Verification items for the finished model (mm, model axes). Round coordinates to 2 decimals unless told otherwise and drop trailing zeros. Order: outer loops, then holes, each group sorted by start corner. A loop starts at its lowest first (then second) coordinate and runs counter-clockwise, first axis right, second up. Notation, with made-up numbers: (-27, 8.25) -> (0, 8.25) arc R25 ccw to (0, 40.25) -> close; hole circle Ø10 at (4, 57). An arc over 180 degrees is marked (long way). Put each result on its own line as item: value.
from build123d import *

# Parameters (mm, degrees)
SKETCH1_R           = 2
SKETCH1_R_2         = 0.75
SKETCH1_R_3         = 0.74964
SKETCH1_W           = 9
SKETCH1_H           = 2.000000357
SKETCH1_W_2         = 5
SKETCH1_H_2         = 2
SKETCH1_W_3         = 8
SKETCH1_H_3         = 6.000000353
SKETCH1_H_4         = 4
SKETCH1_W_4         = 6.000000352
BOSS_EXTRUDE1_DEPTH = 4


with BuildPart() as part:
    # Sketch1 → Boss-Extrude1 (new body)
    with BuildSketch(Plane.XY):
        with BuildLine():
            Line((-12.978641063, -17.999999648), (-12.978641063, -24))
            Line((-12.978641063, -24), (23.021361236, -24))
            Line((23.021361236, -24), (23.021361236, -17.999999648))
            ThreePointArc((23.021361236, -17.999999648), (32.577630228, -15.139859344), (38.991305368, -7.5))
            ThreePointArc((38.991305368, -7.5), (45.219254131, 9.097839331), (47.3354431, 26.698900677))
            ThreePointArc((47.3354431, 26.698900677), (46.554459277, 46.942107237), (44.216150624, 67.064971353))
            Line((44.216150624, 67.064971353), (28.143849376, 69.095028647))
            Line((28.143849376, 69.095028647), (26.638766331, 75.523635508))
            Line((26.638766331, 75.523635508), (10.441233669, 75.806364492))
            Line((10.441233669, 75.806364492), (8.1, 82.51))
            Line((8.1, 82.51), (-8.1, 82.51))
            Line((-8.1, 82.51), (-14.491235706, 82.281481113))
            Line((-14.491235706, 82.281481113), (-30.688764294, 81.998518887))
            ThreePointArc((-30.688764294, 81.998518887), (-37.914532987, 47.276776451), (-37.052658257, 11.821617405))
            ThreePointArc((-37.052658257, 11.821617405), (-29.143237496, -6.421257936), (-12.978641063, -17.999999648))
        make_face()
        with Locations((38.147341743, 11.821617405)):
            Circle(SKETCH1_R, mode=Mode.SUBTRACT)
        with Locations((-14, -9.124358764)):
            Circle(SKETCH1_R, mode=Mode.SUBTRACT)
        with Locations((-5.25, 80.01)):
            Circle(SKETCH1_R_2, mode=Mode.SUBTRACT)
        with Locations((-31.681501662, 43.456405989)):
            Circle(SKETCH1_R, mode=Mode.SUBTRACT)
        with Locations((5.25, 80.01)):
            Circle(SKETCH1_R_2, mode=Mode.SUBTRACT)
        with Locations((5.25, 74.01)):
            Circle(SKETCH1_R_2, mode=Mode.SUBTRACT)
        with Locations((-5.25, 74.01)):
            Circle(SKETCH1_R_2, mode=Mode.SUBTRACT)
        with Locations((-27.795567347, 79.548639007)):
            Circle(SKETCH1_R_2, mode=Mode.SUBTRACT)
        with Locations((-17.297097199, 79.732041708)):
            Circle(SKETCH1_R_2, mode=Mode.SUBTRACT)
        with Locations((-27.690766522, 73.549554345)):
            Circle(SKETCH1_R_2, mode=Mode.SUBTRACT)
        with Locations((-17.192296374, 73.732957046)):
            Circle(SKETCH1_R_2, mode=Mode.SUBTRACT)
        with Locations((23.640854945, 67.074669457)):
            Circle(SKETCH1_R_2, mode=Mode.SUBTRACT)
        with Locations((13.142454146, 67.257919725)):
            Circle(SKETCH1_R_2, mode=Mode.SUBTRACT)
        with Locations((23.745569383, 73.073755628)):
            Circle(SKETCH1_R_2, mode=Mode.SUBTRACT)
        with Locations((13.247168584, 73.257005896)):
            Circle(SKETCH1_R_2, mode=Mode.SUBTRACT)
        with Locations((29.906230336, 60.30489137)):
            Circle(SKETCH1_R_3, mode=Mode.SUBTRACT)
        with Locations((41.075335698, 64.94181766)):
            Circle(SKETCH1_R_3, mode=Mode.SUBTRACT)
        with Locations((30.658103408, 66.257595536)):
            Circle(SKETCH1_R_3, mode=Mode.SUBTRACT)
        with Locations((40.323462626, 58.989113494)):
            Circle(SKETCH1_R_3, mode=Mode.SUBTRACT)
        with Locations((0, 77.509999822)):
            Rectangle(SKETCH1_W, SKETCH1_H, mode=Mode.SUBTRACT)
        Polygon((-9.666, 24.072257636), (-9.153, 28.953126601), (-23.204098338, 30.429956546), (-22.785984485, 34.408044128), (-30.742159647, 35.244271834), (-31.160273501, 31.266184253), (-34.143839187, 31.579769642), (-34.656839187, 26.698900677), (-31.673273501, 26.385315288), (-32.091387354, 22.407227706), (-24.135212191, 21.571), (-23.717098338, 25.549087581), align=None, mode=Mode.SUBTRACT)
        with BuildLine():
            Line((10.358817838, 63.151218734), (10.358817838, 60.151218734))
            Line((10.358817838, 60.151218734), (8.358817838, 60.151218734))
            ThreePointArc((8.358817838, 60.151218734), (-5.478579327, 61.651218734), (8.358817838, 63.151218734))
            Line((8.358817838, 63.151218734), (10.358817838, 63.151218734))
        make_face(mode=Mode.SUBTRACT)
        with Locations((35.147341743, 56.321617405)):
            Rectangle(SKETCH1_W_2, SKETCH1_H_2, mode=Mode.SUBTRACT)
        with BuildLine():
            Line((-17.84156291, 63.151218734), (-15.84156291, 63.151218734))
            Line((-15.84156291, 63.151218734), (-15.84156291, 60.151218734))
            Line((-15.84156291, 60.151218734), (-17.84156291, 60.151218734))
            ThreePointArc((-17.84156291, 60.151218734), (-31.678960076, 61.651218734), (-17.84156291, 63.151218734))
        make_face(mode=Mode.SUBTRACT)
        Polygon((-27.019482275, 78.062008978), (-18.020783292, 78.219211472), (-17.985849684, 76.219516585), (-26.984548667, 76.06231409), align=None, mode=Mode.SUBTRACT)
        with Locations((-14.054335075, 49.87557619)):
            Rectangle(SKETCH1_W_3, SKETCH1_H_3, mode=Mode.SUBTRACT)
        with Locations((17.86306514, 56.321617405)):
            Rectangle(SKETCH1_W_2, SKETCH1_H_2, mode=Mode.SUBTRACT)
        with Locations((-0.478579327, 71.151218734)):
            Rectangle(SKETCH1_W_2, SKETCH1_H_2, mode=Mode.SUBTRACT)
        Polygon((13.970875746, 71.744145048), (13.935970927, 69.744449301), (22.934600183, 69.587377643), (22.969505002, 71.58707339), align=None, mode=Mode.SUBTRACT)
        with BuildLine():
            Line((8.025667975, 48.321617405), (6.025667975, 48.321617405))
            Line((6.025667975, 48.321617405), (6.025667975, 45.321617405))
            Line((6.025667975, 45.321617405), (8.025667975, 45.321617405))
            ThreePointArc((8.025667975, 45.321617405), (21.86306514, 46.821617405), (8.025667975, 48.321617405))
        make_face(mode=Mode.SUBTRACT)
        Polygon((40.143636572, 63.54758064), (31.213865999, 64.675480473), (30.963241642, 62.691245751), (39.893012214, 61.563345918), align=None, mode=Mode.SUBTRACT)
        with BuildLine():
            Line((29.309944577, 45.321617405), (31.309944577, 45.321617405))
            ThreePointArc((31.309944577, 45.321617405), (45.147341743, 46.821617405), (31.309944577, 48.321617405))
            Line((31.309944577, 48.321617405), (29.309944577, 48.321617405))
            Line((29.309944577, 48.321617405), (29.309944577, 45.321617405))
        make_face(mode=Mode.SUBTRACT)
        with Locations((-22.678960076, 71.151218734)):
            Rectangle(SKETCH1_W_2, SKETCH1_H_2, mode=Mode.SUBTRACT)
        Polygon((-4, -2.5), (0, -2.5), (0, 0), (12, 0), (12, -2.5), (16, -2.5), (16, -12.5), (12, -12.5), (12, -15), (0, -15), (0, -12.5), (-4, -12.5), align=None, mode=Mode.SUBTRACT)
        with Locations((-24.554335075, 51.875576367)):
            Rectangle(SKETCH1_W_2, SKETCH1_H_2, mode=Mode.SUBTRACT)
        with Locations((-14.054335075, -0.124358764)):
            Rectangle(SKETCH1_W_3, SKETCH1_H_4, mode=Mode.SUBTRACT)
        with Locations((-24.554335075, -1.124358764)):
            Rectangle(SKETCH1_W_2, SKETCH1_H_2, mode=Mode.SUBTRACT)
        Polygon((0, 23.754659123), (-3, 23.754659123), (-4.5, 21.156582912), (-3, 18.5585067), (0, 18.5585067), (1.5, 21.156582912), align=None, mode=Mode.SUBTRACT)
        with Locations((-2.036620161, 8.717005814)):
            Rectangle(SKETCH1_W_4, SKETCH1_H_4, mode=Mode.SUBTRACT)
        with Locations((-2.036620161, 33.335566927)):
            Rectangle(SKETCH1_W_4, SKETCH1_H_4, mode=Mode.SUBTRACT)
        with Locations((-24.554335075, 8.717005814)):
            Rectangle(SKETCH1_W_2, SKETCH1_H_4, mode=Mode.SUBTRACT)
        with Locations((-24.554335075, 40.727245232)):
            Rectangle(SKETCH1_W_2, SKETCH1_H_4, mode=Mode.SUBTRACT)
    extrude(amount=BOSS_EXTRUDE1_DEPTH)


solid = part.part
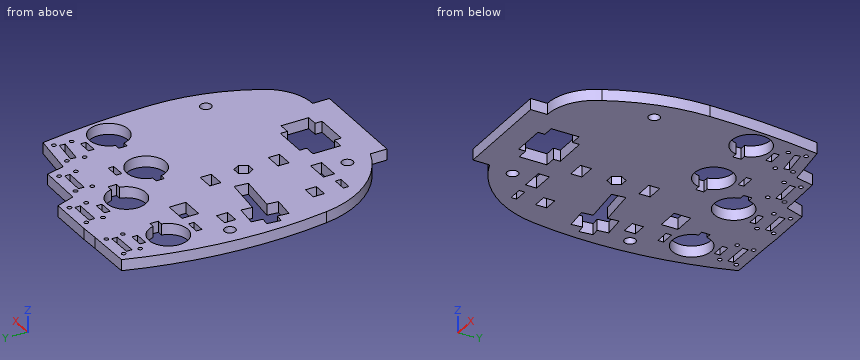
Item 1: Section check B-B on y = 3. Record the boundary of the cut face in (x, z).
Check sheet entries:
outline: (-34.69, 0) -> (43.45, 0) -> (43.45, 4) -> (-34.69, 4) -> close
Item 2: Gauge pin test, flat ends, axial feed: pin 1 Ø2 at (x, z) = (30.5, 1) entering from +Y; pin 2 Ø2 at (y, z) = (46, 2) entering from +X; pin 3 Ø1.2 at (y, z) = (33.5, 2.5) entering from +X. Record the tip position at first contact, or that the pin passes through.
Check sheet entries:
pin 1: stops at y = 68.92
pin 2: stops at x = 46.7
pin 3: stops at x = 47.26
Item 3: Material ranges on L1, parallel to X at y = 22.5, z = 0.2; L2, parallel to Y at x = -27.5, z = 1.2; L3, parallel to X at y = 63, z = 0.65, recorded low to high. Write a range as [from, to].
Check sheet entries:
L1: x = [-38.17, -32.08], [-24.04, -3.72], [0.72, 47.22]
L2: y = [-8.32, 21.92], [34.9, 55.24], [68.06, 72.82], [74.27, 78.86], [80.24, 82.05]
L3: x = [-35.67, -31.55], [-15.84, -5.35], [10.36, 31], [40.07, 44.82]
Item 4: Section check A-A on z = 2.55. State how many separate pieces and enclosed holes the cut face has, then the cut area to 3 significant figures.
Check sheet entries:
separate pieces: 1
enclosed holes: 42
area: 6,280 mm^2
